Build history of the part. All positions in model axes, mm. Give positions to 0.01 mm unless a question says otherwise; leave off trailing zeros. Loops run counter-clockwise (first coordinate to the right, second up) from the corner with the lowest first, then second, coordinate; pieces in that order, holes last. Notation, with made-up numbers: (-27, 30.25) -> (24, 30.25) arc R35 cw to (24, 69.25) -> close; hole circle Ø11 at (-18, 48.25). An arc over 180 degrees is marked (long way). Answer as a JSON object with one key per item and string values. Group by question number.
from build123d import *

# Parameters (mm, degrees)
SKETCH3_R          = 20
CUT_EXTRUDE1_DEPTH = 144.809318196
SKETCH4_R          = 2.5
CUT_EXTRUDE3_DEPTH = 144.809318196
SKETCH5_R          = 26
SKETCH5_R_2        = 24
CUT_EXTRUDE4_DEPTH = 1


with BuildPart() as part:
    # Sketch2 → Revolve1 (revolve)
    with BuildSketch(Plane(origin=(0, 0, 0), x_dir=(0, 0, -1), z_dir=(1, 0, 0)), mode=Mode.PRIVATE) as revolve1_sk:
        Polygon((0, 0), (0, 101.6), (4, 101.6), (4, 95.25), (6, 95.25), (6, 0), align=None)
    revolve(revolve1_sk.sketch.rotate(Axis((0, 0, -6), (0, 0, 1)), 90), axis=Axis((0, 0, -6), (0, 0, 1)))

    # Sketch3 → Cut-Extrude1 (cut, through all)
    with BuildSketch(Plane.XY):
        with Locations((-20, 0)):
            Circle(SKETCH3_R)
    extrude(amount=-CUT_EXTRUDE1_DEPTH, mode=Mode.SUBTRACT)

    # Sketch4 → Cut-Extrude3 (cut, through all)
    with BuildSketch(Plane.XY):
        with Locations((-20, 30)):
            Circle(SKETCH4_R)
        with Locations((5.980762114, 15)):
            Circle(SKETCH4_R)
        with Locations((5.980762114, -15)):
            Circle(SKETCH4_R)
        with Locations((-20, -30)):
            Circle(SKETCH4_R)
        with Locations((-45.980762114, -15)):
            Circle(SKETCH4_R)
        with Locations((-45.980762114, 15)):
            Circle(SKETCH4_R)
    extrude(amount=-CUT_EXTRUDE3_DEPTH, mode=Mode.SUBTRACT)

    # Sketch5 → Cut-Extrude4 (cut)
    with BuildSketch(Plane.XY):
        with Locations((-20, 0)):
            Circle(SKETCH5_R)
        with Locations((-20, 0)):
            Circle(SKETCH5_R_2, mode=Mode.SUBTRACT)
    extrude(amount=-CUT_EXTRUDE4_DEPTH, mode=Mode.SUBTRACT)


solid = part.part
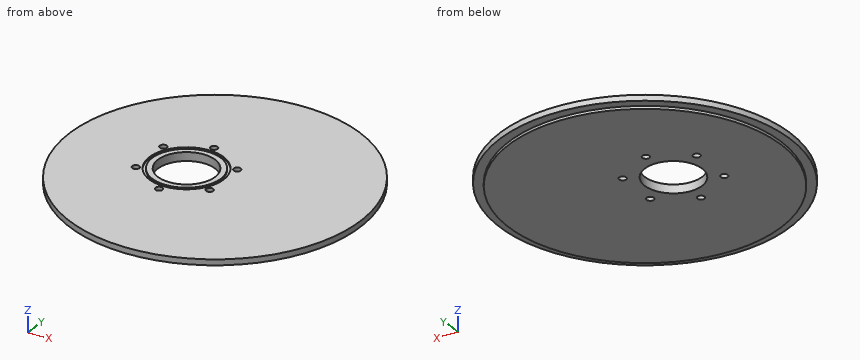
(1) Saw through at D-D on x = -77. List the corners of the cut face in (y, z), plus the area to 3 significant figures.
(2) Saw through at A-A on x = -6. List the corners of the cut face in (y, z).
(3) Saw through at C-C on y = -30. List the corners of the cut face in (x, z), plus the area to 3 significant figures.
(4) Probe line 1 along Y through (x, z) = (-20, -1.45); line 2 along Y through (x, z) = (-20, -4.65); line 3 along Y through (x, z) = (-45.5, -2.6). List the from-to ranges inside material, lowest first. Write a range as [from, to].
(5) Saw through at B-B on y = 15. List the corners of the cut face in (x, z) (3 decimals).
(6) Pin check, flat tip, straight feed: pin 1 (1.5 mm diameter, centred on y = 51, z = -3, fed in from -X). Stop position of the tip, or through.
Calculated:
{
 "1": {"outline": "(-66.28, -4) -> (-56.07, -4) -> (-56.07, -6) -> (56.07, -6) -> (56.07, -4) -> (66.28, -4) -> (66.28, 0) -> (-66.28, 0) -> close", "area": "755 mm^2"},
 "2": {"outline": "(-101.42, -4) -> (-95.06, -4) -> (-95.06, -6) -> (-14.28, -6) -> (-14.28, 0) -> (-19.49, 0) -> (-19.49, -1) -> (-21.91, -1) -> (-21.91, 0) -> (-101.42, 0) -> close; (14.28, -6) -> (95.06, -6) -> (95.06, -4) -> (101.42, -4) -> (101.42, 0) -> (21.91, 0) -> (21.91, -1) -> (19.49, -1) -> (19.49, 0) -> (14.28, 0) -> close"},
 "3": {"outline": "(-97.07, -4) -> (-90.4, -4) -> (-90.4, -6) -> (-22.5, -6) -> (-22.5, 0) -> (-97.07, 0) -> close; (-17.5, -6) -> (90.4, -6) -> (90.4, -4) -> (97.07, -4) -> (97.07, 0) -> (-17.5, 0) -> close", "area": "1,110 mm^2"},
 "4": {"line 1": "y = [-99.61, -32.5], [-27.5, -20], [20, 27.5], [32.5, 99.61]", "line 2": "y = [-93.13, -32.5], [-27.5, -20], [20, 27.5], [32.5, 93.13]", "line 3": "y = [-90.84, -17.45], [-12.55, 12.55], [17.45, 90.84]"},
 "5": {"outline": "(-100.487, -4) -> (-94.061, -4) -> (-94.061, -6) -> (-48.481, -6) -> (-48.481, 0) -> (-100.487, 0) -> close; (-43.481, -6) -> (-33.229, -6) -> (-33.229, 0) -> (-38.735, 0) -> (-38.735, -1) -> (-41.237, -1) -> (-41.237, 0) -> (-43.481, 0) -> close; (-6.771, -6) -> (3.481, -6) -> (3.481, 0) -> (1.237, 0) -> (1.237, -1) -> (-1.265, -1) -> (-1.265, 0) -> (-6.771, 0) -> close; (8.481, -6) -> (94.061, -6) -> (94.061, -4) -> (100.487, -4) -> (100.487, 0) -> (8.481, 0) -> close"},
 "6": {"pin 1": "stops at x = -88.3"}
}
